```python
from build123d import *

# Parameters (mm, degrees)
F0_R         = 1.575
F0_R_2       = 13.5
F0_W         = 5
F0_H         = 21.15
F1_DEPTH     = 2
F2_DEPTH     = 20
F3_DEPTH     = 16
F4_R         = 6.05
F5_DEPTH     = 2.5
F6_W         = 6.1
F6_H         = 12
F7_DEPTH     = 18.5
F8_W         = 3
F8_H         = 12
F9_DEPTH     = 12
F10_T1_DEPTH = 2
F10_T3_DEPTH = 26.125
F10_T5_DEPTH = 37.75
F10_T7_DEPTH = 17.75
F10_T9_DEPTH = 5.4173756904
F11_R        = 1.49999
F12_SIZE     = 5
F13_SIZE2    = 16
F13_SIZE     = 10
F14_R        = 5


# Not quite as in the source:
# - a fillet or chamfer that OpenCascade refuses, or shapes differently, is made with other operations: its cross-section is extruded or revolved along the edge and cut away or added
# - a fillet or chamfer is up to 0.001 mm smaller than in the source, because OpenCascade refuses the exact size
# - a feature names something its author has since deleted; it is built from what else it names


with BuildPart() as f1:
    # F0 (on Front) → F1 (new body)
    with BuildSketch(Plane.XZ):
        Polygon((-21.15, -17.0841360082), (-21.15, 0), (-25.15, 0), (-25.15, -25.15), (-7.15, -25.15), (-7.15, -21.15), (-17.0841360082, -21.15), (-21.15, -21.15), align=None)
        Polygon((21.15, 17.0841360082), (17.0841360082, 21.15), (-17.0841360082, 21.15), (-21.15, 17.0841360082), (-21.15, 0), (-21.15, -17.0841360082), (-17.0841360082, -21.15), (-7.15, -21.15), (0, -21.15), (21.15, -21.15), (21.15, 0), align=None)
        with Locations((-15.5, -15.5)):
            Circle(F0_R, mode=Mode.SUBTRACT)
        with Locations((15.5, -15.5)):
            Circle(F0_R, mode=Mode.SUBTRACT)
        Circle(F0_R_2, mode=Mode.SUBTRACT)
        with Locations((-15.5, 15.5)):
            Circle(F0_R, mode=Mode.SUBTRACT)
        with Locations((15.5, 15.5)):
            Circle(F0_R, mode=Mode.SUBTRACT)
        Polygon((-17.0841360082, -21.15), (-21.15, -17.0841360082), (-21.15, -21.15), align=None)
        Polygon((26.15, -21.15), (21.15, -21.15), (0, -21.15), (21.1919918656, -31.15), (26.15, -31.15), align=None)
        Polygon((28.65, 0), (26.15, 0), (26.15, -21.15), (26.15, -31.15), (46.65, -31.15), (46.65, -28.65), (28.65, -28.65), align=None)
        with Locations((23.65, -10.575)):
            Rectangle(F0_W, F0_H)
    extrude(amount=F1_DEPTH)

    # F0 (on Front) → F2 (join)
    with BuildSketch(Plane.XZ):
        Polygon((-21.15, -17.0841360082), (-21.15, 0), (-25.15, 0), (-25.15, -25.15), (-7.15, -25.15), (-7.15, -21.15), (-17.0841360082, -21.15), (-21.15, -21.15), align=None)
        Polygon((-17.0841360082, -21.15), (-21.15, -17.0841360082), (-21.15, -21.15), align=None)
    extrude(amount=F2_DEPTH)

    # F0 (on Front) → F3 (join)
    with BuildSketch(Plane.XZ):
        Polygon((28.65, 0), (26.15, 0), (26.15, -21.15), (26.15, -31.15), (46.65, -31.15), (46.65, -28.65), (28.65, -28.65), align=None)
    extrude(amount=F3_DEPTH)

    # F4 (on face) → F5 (cut, through all)
    with BuildSketch(Plane.XY.offset(-28.65)):
        with Locations((38.65, -8)):
            Circle(F4_R)
    extrude(amount=-F5_DEPTH, mode=Mode.SUBTRACT)

    # F6 (on face) → F7 (join)
    with BuildSketch(Plane(origin=(0, 0, -25.15), x_dir=(1, 0, 0), z_dir=(0, 0, -1))):
        with Locations((-10.2, 14)):
            Rectangle(F6_W, F6_H)
    extrude(amount=F7_DEPTH)

    # F8 (on face) → F9 (cut, through all)
    with BuildSketch(Plane.XZ.offset(20)):
        with Locations((-10.2, -35.15)):
            Rectangle(F8_W, F8_H)
    extrude(amount=-F9_DEPTH, mode=Mode.SUBTRACT)

    # F10: fillet of radius 3.05 on 8 edges, made by hand

    # F10_s2 → F10_t1 (join)
    with BuildSketch(Plane.XZ):
        with BuildLine():
            ThreePointArc((-0.6834751381, -21.15), (-0.0165404304, -21.2238114818), (0.6181139894, -21.4416733799))
            Line((0.6181139894, -21.4416733799), (0, -21.15))
            Line((0, -21.15), (-0.6834751381, -21.15))
        make_face()
    extrude(amount=F10_T1_DEPTH)

    # F10_s4 → F10_t3 (cut)
    with BuildSketch(Plane.XY.offset(-51.275)):
        with BuildLine():
            ThreePointArc((-13.25, -11.05), (-12.3566756826, -8.8933243174), (-10.2, -8))
            Line((-10.2, -8), (-13.25, -8))
            Line((-13.25, -8), (-13.25, -11.05))
        make_face()
        with BuildLine():
            ThreePointArc((-7.15, -11.05), (-8.0433243174, -8.8933243174), (-10.2, -8))
            Line((-10.2, -8), (-7.15, -8))
            Line((-7.15, -8), (-7.15, -11.05))
        make_face()
        with BuildLine():
            ThreePointArc((-10.2, -20), (-12.3566756826, -19.1066756826), (-13.25, -16.95))
            Line((-13.25, -16.95), (-13.25, -20))
            Line((-13.25, -20), (-10.2, -20))
        make_face()
    extrude(amount=F10_T3_DEPTH, mode=Mode.SUBTRACT)

    # F10_s6 → F10_t5 (cut)
    with BuildSketch(Plane.XY.offset(-51.275)):
        with BuildLine():
            ThreePointArc((-10.2, -20), (-8.0433243174, -19.1066756826), (-7.15, -16.95))
            Line((-7.15, -16.95), (-7.15, -20))
            Line((-7.15, -20), (-10.2, -20))
        make_face()
    extrude(amount=F10_T5_DEPTH, mode=Mode.SUBTRACT)

    # F10_s8 → F10_t7 (cut)
    with BuildSketch(Plane.XY.offset(-38.775)):
        with BuildLine():
            ThreePointArc((46.65, -12.95), (45.7566756826, -15.1066756826), (43.6, -16))
            Line((43.6, -16), (46.65, -16))
            Line((46.65, -16), (46.65, -12.95))
        make_face()
        with BuildLine():
            ThreePointArc((43.6, 0), (45.7566756826, -0.8933243174), (46.65, -3.05))
            Line((46.65, -3.05), (46.65, 0))
            Line((46.65, 0), (43.6, 0))
        make_face()
    extrude(amount=F10_T7_DEPTH, mode=Mode.SUBTRACT)

    # F10_s10 → F10_t9 (cut)
    with BuildSketch(Plane.XZ.offset(-1.7086878452)):
        with BuildLine():
            ThreePointArc((20.5738778763, -30.8583266201), (21.208532296, -31.0761885182), (21.8754670037, -31.15))
            Line((21.8754670037, -31.15), (21.1919918656, -31.15))
            Line((21.1919918656, -31.15), (20.5738778763, -30.8583266201))
        make_face()
    extrude(amount=F10_T9_DEPTH, mode=Mode.SUBTRACT)

    # F11 (radius 1.5 in the source; OpenCascade refuses exactly that, so slightly less here)
    f11_edges = [f1.edges().sort_by_distance(p)[0] for p in [
        (-11.7, -14, -29.15),
        (-8.7, -14, -29.15),
        (-11.7, -14, -41.15),
        (-8.7, -14, -41.15),
    ]]
    fillet(f11_edges, radius=F11_R)

    # F12
    f12_edges = [f1.edges().sort_by_distance(p)[0] for p in [
        (-25.15, -10, -25.15),
    ]]
    chamfer(f12_edges, length=F12_SIZE)

    # F13
    f13_edges = [f1.edges().sort_by_distance(p)[0] for p in [
        (27.4, -16, 0),
    ]]
    f13_side = f1.faces().sort_by_distance((26.65, -6.6, 0))[0]
    chamfer(f13_edges, length=F13_SIZE, length2=F13_SIZE2, reference=f13_side)

    # F14
    f14_edges = [f1.edges().sort_by_distance(p)[0] for p in [
        (27.4, -16, -16),
        (27.4, -6, 0),
    ]]
    fillet(f14_edges, radius=F14_R)


solid = f1.part
```
CAD build for the part. Positions are in the model's coordinates, mm. A direction names the side the tool comes from. Round coordinates to 2 decimals unless told otherwise and drop trailing zeros. Loops run counter-clockwise (first coordinate to the right, second up) from the corner with the lowest first, then second, coordinate; pieces in that order, holes last. Notation, with made-up numbers: M 6.25,25.25 L 19.25,25.25 A21 cw 19.25,43.25 Z; hole C 32,28 d11. An arc over 180 degrees is marked long. Return JSON: item names as keys, results as strings. Group by question number.
(1) Mould opens along Z. For faces 1 (the cylindrical face through (-14.045, -0.986, 14.897)), 2 (the flat face through (31, -8, -31.15)), 3 (the flat face through (13, -2, -5)) say: +Z half, -Z half, draft (parallel to the pull), parting line (faces both ways), or undercut.
(2) Saw through at C-C, the plane y = -6.25. List the corners of the cut face in (x, z).
(3) Wall check: probe 1 along X at (y, z) = (-5.75, -3.5); probe 2 along Z at (x, y) = (15.5, -0.5) (3 decimals); probe 3 along Y at (x, z) = (22, -20). Give the ranges that are in metal, low to high. Write a range as [from, to].
(4) Saw through at D-D, the plane x = 3. List the corners of the cut face in (y, z), and give its area (3 significant figures).
(5) Saw through at B-B, the plane x = -15.5. List the corners of the cut face in (y, z) (3 decimals), and give its area (3 significant figures).
(6) Tool access for faces 4 (the flat face through (26.15, -7, -19)), 5 (the flat face through (27.417, -11.409, -8.654)), 6 (the cylindrical face through (-9.15, -13.92, -29.58)), 7 (the flat face through (25, -1, 0)): list every direction of +Z, -Z, +X, -X, +Y, -Y with a clear straight run to the whole face (end or side of a thin tool).
(7) Drop flat-ended pins along their axis: P1, Ø2, axis at y = -16.5, z = -32.5, coming from the +X side; P2, Ø4, axis at x = 20, y = -3, coming from the +Z side; P3, Ø11, axis at x = -9.5, y = -10, coming from the +Z side; P4, Ø3.5, axis at x = 15.5, z = 15.5, coming from the +Y side. Give the stop position or say it passes through.
(8) Saw through at A-A, the plane z = 15.5. List the corners of the cut face in (x, y) (3 decimals), and give its area (3 significant figures).
Answer list:
{
 "1": {"face 1": "undercut", "face 2": "-Z half", "face 3": "draft"},
 "2": {"outline": "M -25.15,-20.15 L -20.15,-25.15 L -7.15,-25.15 L -7.15,-21.15 L -17.08,-21.15 L -21.15,-17.08 L -21.15,0 L -25.15,0 Z; M 26.15,-31.15 L 32.86,-31.15 L 32.86,-28.65 L 28.65,-28.65 L 28.65,-1.02 L 26.15,-1.02 Z; M 44.44,-31.15 L 46.65,-31.15 L 46.65,-28.65 L 44.44,-28.65 Z"},
 "3": {"probe 1": "[-25.15, -21.15], [26.15, 28.65]", "probe 2": "[-28.464, -17.075], [-13.925, 13.925], [17.075, 21.15]", "probe 3": "[-2, 0]"},
 "4": {"outline": "M -2,-22.57 L 0,-22.57 L 0,-13.16 L -2,-13.16 Z; M -2,13.16 L 0,13.16 L 0,21.15 L -2,21.15 Z", "area": "34.8 mm2"},
 "5": {"outline": "M -20,-25.15 L 0,-25.15 L 0,-17.075 L -2,-17.075 L -2,-21.15 L -20,-21.15 Z; M -2,-13.925 L 0,-13.925 L 0,13.925 L -2,13.925 Z; M -2,17.075 L 0,17.075 L 0,21.15 L -2,21.15 Z", "area": "152 mm2"},
 "6": {"face 4": "+Z, -Z, -Y", "face 5": "+Z, +X, -Y", "face 6": "+Y, -Y", "face 7": "+Z, +X, +Y, -Y"},
 "7": {"P1": "x = -7.15", "P2": "z = 19.97", "P3": "z = -21.15", "P4": "y = 0"},
 "8": {"outline": "M -21.15,-2 L -17.075,-2 L -17.075,0 L -21.15,0 Z; M -13.925,-2 L 13.925,-2 L 13.925,0 L -13.925,0 Z; M 17.075,-2 L 21.15,-2 L 21.15,0 L 17.075,0 Z", "area": "72.0 mm2"}
}
